Autodesk Inventor part; units mm, degrees
ref_plane "YZ Plane" through (0, 0, 0) normal (1, 0, 0) x (0, 1, 0)
ref_plane "XZ Plane" through (0, 0, 0) normal (0, 1, 0) x (-1, 0, 0)
ref_plane "XY Plane" through (0, 0, 0) normal (0, 0, 1) x (1, 0, 0)
sketch "Sketch1" plane through (0, 0, 0) normal (0, 0, 1) x (1, 0, 0)
  circle A0 centre (0, 0) radius 24.9555
  circle A1 centre (0, 0) radius 7.3025
  dimension "d0" = 49.911
  dimension "d2" = 14.605
extrude "Extrusion1" add sketch "Sketch1" along normal blind 3.937
sketch "Sketch2" plane through (0, 0, 3.937) normal (0, 0, 1) x (1, 0, 0)
  circle A0 centre (0, 0) radius 7.3025
  circle A1 centre (0, 0) radius 12.7
  dimension "d5" = 25.4
extrude "Extrusion2" add sketch "Sketch2" along normal blind 6.35
chamfer "Chamfer1" distance 1.524 angle 45 1 edges at (-24.9555, 0, 3.937)
chamfer "Chamfer2" distance 1.524 angle 45 1 edges at (-24.9555, 0, 0)
properties part number "Sprocket Large"
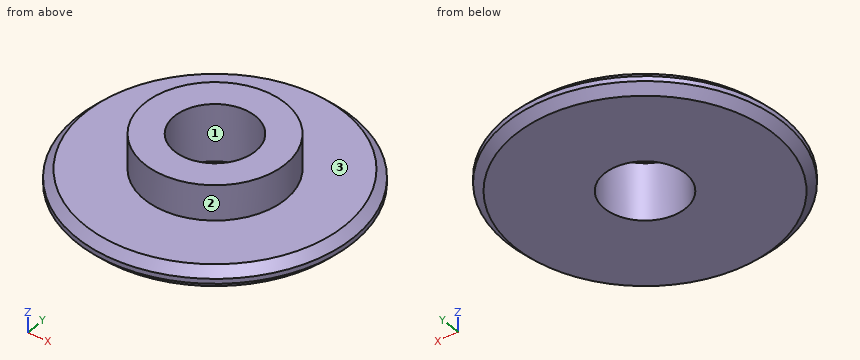
CAD build for the part. Positions are in the model's coordinates, mm. Face numbers are marked on the shaded views. Coordinates: 2 decimals unless noted, no trailing zeros. Loops run counter-clockwise (first coordinate to the right, second up) from the corner with the lowest first, then second, coordinate; pieces in that order, holes last. Notation, with made-up numbers: (88.5, -24) - (101.5, -24) arc R28 cw to (101.5, 3) - close; hole circle Ø7 at (32, -30.5). An arc over 180 degrees is marked (long way). Write item = value, one per line. Start each with the question number.
Q1. Flat gauge pins, fed straight in: pin 1 Ø5 at (y, z) = (10, 7.5) entering from +X; pin 2 Ø4 at (x, z) = (2.5, 2) entering from +Y; pin 3 Ø4 at (x, z) = (16, 2) entering from -Y. Where does each tip first touch, or does it go through?
Q2. Cut at A-A, the plane y = 0. List the corners of the cut face in (x, z), then the cut area to 3 significant figures.
Q3. Drill centre lines: L1, parallel to Y at x = 0, z = 2.25; L2, parallel to Y at x = 0, z = 8.25; L3, parallel to Z at x = -20, y = 9. Where is each one in solid material? Low to high.
Q4. Cut at C-C, the plane z = 9. List the corners of the cut face in (x, y) (1 decimal), then the cut area to 3 significant figures.
Q5. Pull direction X, two halves, no side cores. Call the marked faces 1, 2 and 3: pulls with the +X half, pulls with the -X half, needs draft (parallel to the pull), parting line crosses it, or undercut.
Computed:
q1.pin_1 = 10.25
q1.pin_2 = 24.95
q1.pin_3 = -20.66
q2.outline = (-24.96, 1.52) - (-23.43, 0) - (-7.3, 0) - (-7.3, 10.29) - (-12.7, 10.29) - (-12.7, 3.94) - (-23.43, 3.94) - (-24.96, 2.41) - close; (7.3, 0) - (23.43, 0) - (24.96, 1.52) - (24.96, 2.41) - (23.43, 3.94) - (12.7, 3.94) - (12.7, 10.29) - (7.3, 10.29) - close
q2.area = 203 mm²
q3.L1 = -24.96 to -7.3, 7.3 to 24.96
q3.L2 = -12.7 to -7.3, 7.3 to 12.7
q3.L3 = 0 to 3.94
q4.outline = circle Ø25.4 at (0, 0); hole circle Ø14.6 at (0, 0)
q4.area = 339 mm²
q5.face_1 = undercut
q5.face_2 = parting line crosses it
q5.face_3 = needs draft
